Check sheet for the modelled part. Datum: model origin and axes. Units: mm. A direction names the side the tool comes from. Round coordinates to 2 decimals unless told otherwise and drop trailing zeros. Loops run counter-clockwise (first coordinate to the right, second up) from the corner with the lowest first, then second, coordinate; pieces in that order, holes last. Notation, with made-up numbers: (61, -20.75) - (94, -20.75) arc R18 ccw to (94, 13.25) - close; hole circle Ø11 at (21, -15.75). An arc over 180 degrees is marked (long way). Put each result on its own line as item: value.
```python
from build123d import *

# Parameters (mm, degrees)
F1_DEPTH = 3
F2_R     = 1.5
F3_DEPTH = 3.001


with BuildPart() as f1:
    # F0 (on Top) → F1 (new body)
    with BuildSketch(Plane.XY):
        Polygon((-13.195418, -19.596273), (-3.195418, -19.596273), (-3.195418, 7.403542), (-0.345418, 7.403542), (-0.345418, 11.403542), (-15.945418, 11.403542), (-15.945418, 7.403542), (-13.095418, 7.403542), align=None)
    extrude(amount=F1_DEPTH)

    # F2 (on face) → F3 (cut, through all)
    with BuildSketch(Plane.XY.offset(3)):
        with BuildLine():
            Line((-9.695418, 3.499953), (-9.706427, 1.549641))
            Line((-9.706427, 1.549641), (-9.706892, 1.467193))
            ThreePointArc((-9.706892, 1.467193), (-8.307444, 0.003303), (-6.725357, 1.267591))
            Line((-6.725357, 1.267591), (-6.695629, 3.474782))
            ThreePointArc((-6.695629, 3.474782), (-8.182832, 4.999901), (-9.695418, 3.499953))
        make_face()
        with Locations((-8.195418, -14.570472)):
            Circle(F2_R)
    extrude(amount=-F3_DEPTH, mode=Mode.SUBTRACT)


solid = f1.part
```
Item 1: Section check B-B on y = 0.5. Enter the section's corners in (x, z), then the cut area to 3 significant figures.
Filled sheet:
outline: (-13.12, 0) - (-9.33, 0) - (-9.33, 3) - (-13.12, 3) - close; (-7.09, 0) - (-3.2, 0) - (-3.2, 3) - (-7.09, 3) - close
area: 23.1 mm²
Item 2: Tool access check on faces 4 (the cylindrical face through (-8.338, 0.006, 1.521)), 5 (the flat face through (-8, -4, 0)), 6 (the flat face through (-3.195, -6, 1)). Record the directions out of +Z, -Z, +X, -X, +Y, -Y that give a thin tool (end or side, any length) a straight path to the whole face; none if there is none.
Filled sheet:
face 4: +Z, -Z
face 5: -Z, +X, -X, +Y, -Y
face 6: +Z, -Z, +X, -Y
Item 3: Section check C-C on x = -14.25. Enter the section's corners in (y, z).
Filled sheet:
outline: (7.4, 0) - (11.4, 0) - (11.4, 3) - (7.4, 3) - close
Item 4: Release check for a two-part mould opening along X. For faces 1 (the flat face through (-8, -4, 3)), 2 (the cylindrical face through (-8.15, 5, 1.52)), 3 (the flat face through (-15.945, 9, 1)) record: +X half, -X half, draft (parallel to the pull), parting line (faces both ways), or undercut.
Filled sheet:
face 1: draft
face 2: undercut
face 3: -X half
Item 5: Go/stop test with flat-tipped pins: pin 1 (3 mm diameter, centred on x = -6.5, y = 3.5, fed in from -Z); pin 2 (0.9 mm diameter, centred on y = -3.5, z = 2, fed in from +X); pin 3 (1.4 mm diameter, centred on x = -1.5, z = 2, fed in from -Y). Record where each tip stops, or that it passes through.
Filled sheet:
pin 1: z = 0
pin 2: x = -3.2
pin 3: y = 7.4
Item 6: Thickness scan on line 1 (Y direction, x = -8.25, z = 0.25); line 2 (X direction, y = 6, z = 0.2); line 3 (Y direction, x = -7.5, z = 2.85). Record the ranges inside material, lowest first. Write a range as from..to.
Filled sheet:
line 1: -19.6..-16.07, -13.07..0, 5..11.4
line 2: -13.1..-3.2
line 3: -19.6..-15.9, -13.24..0.18, 4.83..11.4
Item 7: Section check A-A on z = 0.85. Enter the section's corners in (x, y), then the cut area to 3 significant figures.
Filled sheet:
outline: (-15.95, 7.4) - (-13.1, 7.4) - (-13.2, -19.6) - (-3.2, -19.6) - (-3.2, 7.4) - (-0.35, 7.4) - (-0.35, 11.4) - (-15.95, 11.4) - close; hole (-9.71, 1.47) arc R1.5 ccw to (-6.73, 1.27) - (-6.7, 3.47) arc R1.5 ccw (long way) to (-9.7, 3.5) - (-9.71, 1.55) - close; hole circle Ø3 at (-8.2, -14.57)
area: 311 mm²
Item 8: Section check D-D on y = -8. Enter the section's corners in (x, z).
Filled sheet:
outline: (-13.15, 0) - (-3.2, 0) - (-3.2, 3) - (-13.15, 3) - close
